from build123d import *

# Parameters (mm, degrees)
F0_W     = 100
F0_H     = 50
F1_DEPTH = 20
F2_R     = 5
F3_T     = -2.5


with BuildPart() as f1:
    # F0 (on Top) → F1 (new body)
    with BuildSketch(Plane.XY):
        Rectangle(F0_W, F0_H)
    extrude(amount=F1_DEPTH)

    # F2
    f2_edges = [f1.edges().sort_by_distance(p)[0] for p in [
        (-50, 0, 20),
        (0, -25, 20),
        (50, 0, 20),
        (0, 25, 20),
        (50, 25, 10),
        (50, -25, 10),
        (-50, -25, 10),
        (-50, 25, 10),
    ]]
    fillet(f2_edges, radius=F2_R)

    # F3
    f3_openings = [f1.faces().sort_by_distance(p)[0] for p in [
        (0, 0, 0),
    ]]
    offset(amount=F3_T, openings=f3_openings)

    # F4: F1 across plane


with BuildPart() as f1_1:
    add(f1.part)
    add(f1.part.mirror(Plane.XY))


solid = f1_1.part
The listing builds one solid part. Answer for the finished solid, in the listing's coordinates (mm). A direction names the side the tool comes from. Give positions to 0.01 mm unless a question says otherwise; leave off trailing zeros. Write each loop counter-clockwise with the first axis right and the second up, starting at its lowest first coordinate (ties: lowest second). Pieces come first, ordered by that corner, then holes. Notation, with made-up numbers: (87, 65) -> (108, 65) arc R28 cw to (108, 83) -> close; hole circle Ø4 at (15.5, 19.25). An arc over 180 degrees is marked (long way). Use a Markdown table: item, result.
(1) Section B-B, the plane y = 10 is taken. Determine the outline of the cut face in (x, z).
Return value:
| item | result |
|---|---|
| outline | (-50, -15) arc R5 ccw to (-45, -20) -> (45, -20) arc R5 ccw to (50, -15) -> (50, 15) arc R5 ccw to (45, 20) -> (-45, 20) arc R5 ccw to (-50, 15) -> close; hole (-47.5, -15) arc R2.5 ccw to (-45, -17.5) -> (45, -17.5) arc R2.5 ccw to (47.5, -15) -> (47.5, 15) arc R2.5 ccw to (45, 17.5) -> (-45, 17.5) arc R2.5 ccw to (-47.5, 15) -> close |
(2) Determine the mould class of faces 3 (the cylindrical face through (-46.787, 0.28, 16.748)), 4 (the cylindrical face through (-49, -23, 0)), 5 (the flat face through (-1, 0, -20)) for opening direction X: released by +X, released by -X, zero draft, split by the parting line, or undercut.
Return value:
| item | result |
|---|---|
| face 3 | undercut |
| face 4 | released by -X |
| face 5 | zero draft |
(3) For faces 1 (the flat face through (47.5, 0, 0)), 2 (the cylindrical face through (-49, 23, 0)), determine the directions among +Z, -Z, +X, -X, +Y, -Y from which every point of the face is accessible in a straight line to the end or side of a thin tool.
Return value:
| item | result |
|---|---|
| face 1 | none |
| face 2 | +Z, -Z, -X, +Y |
(4) Section A-A, the plane x = 11.5 is taken. Determine the outline of the cut face in (y, z), then the cut area to 3 significant figures.
Return value:
| item | result |
|---|---|
| outline | (-25, -15) arc R5 ccw to (-20, -20) -> (20, -20) arc R5 ccw to (25, -15) -> (25, 15) arc R5 ccw to (20, 20) -> (-20, 20) arc R5 ccw to (-25, 15) -> close; hole (-22.5, -15) arc R2.5 ccw to (-20, -17.5) -> (20, -17.5) arc R2.5 ccw to (22.5, -15) -> (22.5, 15) arc R2.5 ccw to (20, 17.5) -> (-20, 17.5) arc R2.5 ccw to (-22.5, 15) -> close |
| area | 409 mm2 |
(5) Find the intervals of material crossed by probe 1 along Z at (x, y) = (41, -1.5); probe 2 along Y at (x, z) = (-24, 0.5); probe 3 along X at (y, z) = (15, -12), in increasing order. Write a range as from..to.
Return value:
| item | result |
|---|---|
| probe 1 | -20..-17.5, 17.5..20 |
| probe 2 | -25..-22.5, 22.5..25 |
| probe 3 | -50..-47.5, 47.5..50 |
